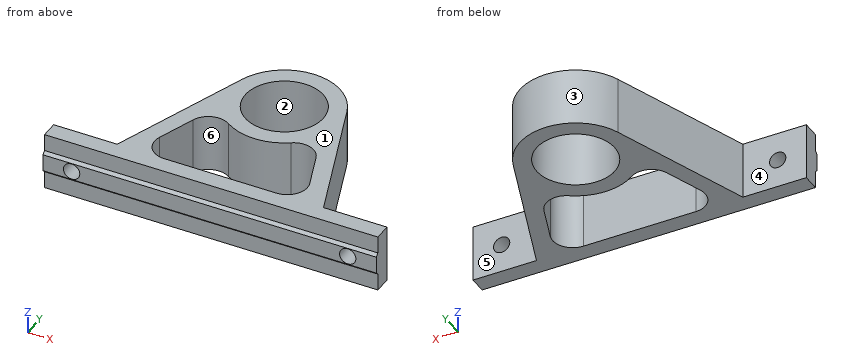
```python
from build123d import *

# Parameters (mm, degrees)
F0_R        = 13.6
F0_W        = 59.3062995352
F0_H        = 6
F1_DEPTH    = 20
F2_R        = 7
F3_W        = 116.4440756161
F3_H        = 2
F4_DEPTH    = 1
F5_T4_DEPTH = 116.4440756161
F5_T9_DEPTH = 116.4440756161
F6_R        = 2.85
F7_DEPTH    = 25


# Not quite as in the source:
# - a fillet or chamfer that OpenCascade refuses, or shapes differently, is made with other operations: its cross-section is extruded or revolved along the edge and cut away or added


with BuildPart() as f1:
    # F0 (on Top) → F1 (new body)
    with BuildSketch(Plane.XY):
        with BuildLine():
            ThreePointArc((17.4985003919, 39.3946247011), (18.9930350082, 43.5824643545), (19.5, 48))
            ThreePointArc((19.5, 48), (19.2037511837, 51.3861394645), (18.3240061053, 54.6693927949))
            ThreePointArc((18.3240061053, 54.6693927949), (0, 67.5), (-18.3240061053, 54.6693927949))
            ThreePointArc((-18.3240061053, 54.6693927949), (-19.4715851439, 46.9476825647), (-17.4985003919, 39.3946247011))
            ThreePointArc((-17.4985003919, 39.3946247011), (0, 28.5), (17.4985003919, 39.3946247011))
        make_face()
        with Locations((0, 48)):
            Circle(F0_R, mode=Mode.SUBTRACT)
        with BuildLine():
            ThreePointArc((-17.4985003919, 39.3946247011), (-19.4715851439, 46.9476825647), (-18.3240061053, 54.6693927949))
            Line((-18.3240061053, 54.6693927949), (-36.0382164025, 6))
            Line((-36.0382164025, 6), (-29.6531497676, 6))
            Line((-29.6531497676, 6), (-17.4985003919, 39.3946247011))
        make_face()
        Polygon((-29.6531497676, 6), (-36.0382164025, 6), (-38.2220378081, 0), (-29.6531497676, 0), align=None)
        Polygon((-38.2220378081, 0), (-36.0382164025, 6), (-58.2220378081, 6), (-58.2220378081, 0), align=None)
        with Locations((0, 3)):
            Rectangle(F0_W, F0_H)
        Polygon((38.2220378081, 0), (36.0382164025, 6), (29.6531497676, 6), (29.6531497676, 0), align=None)
        Polygon((58.2220378081, 6), (36.0382164025, 6), (38.2220378081, 0), (58.2220378081, 0), align=None)
        with BuildLine():
            ThreePointArc((18.3240061053, 54.6693927949), (19.2037511837, 51.3861394645), (19.5, 48))
            ThreePointArc((19.5, 48), (18.9930350082, 43.5824643545), (17.4985003919, 39.3946247011))
            Line((17.4985003919, 39.3946247011), (29.6531497676, 6))
            Line((29.6531497676, 6), (36.0382164025, 6))
            Line((36.0382164025, 6), (18.3240061053, 54.6693927949))
        make_face()
    extrude(amount=F1_DEPTH)

    # F2
    f2_edges = [f1.edges().sort_by_distance(p)[0] for p in [
        (-17.4985, 39.394625, 10),
        (17.4985, 39.394625, 10),
        (-29.65315, 6, 10),
        (29.65315, 6, 10),
    ]]
    fillet(f2_edges, radius=F2_R)

    # F3 (on face) → F4 (join)
    with BuildSketch(Plane.XZ):
        with Locations((0, 10)):
            Rectangle(F3_W, F3_H)
    extrude(amount=F4_DEPTH)

    # F5: chamfer of 3 on 2 edges, made by hand


with BuildPart() as f5_tool2:
    # F5_s3 → F5_t4 (new body)
    with BuildSketch(Plane.YZ.offset(58.2220378081)):
        Polygon((0, 14), (-3, 11), (0, 11), align=None)
    extrude(amount=-F5_T4_DEPTH)

    split(bisect_by=Plane.XZ.offset(1), keep=Keep.BOTTOM)


with BuildPart() as f1_1:
    add(f1.part)

    # F5_t1: union F5_tool2
    add(f5_tool2.part)


with BuildPart() as f5_tool7:
    # F5_s8 → F5_t9 (new body)
    with BuildSketch(Plane.YZ.offset(-58.2220378081)):
        Polygon((0, 6), (-3, 9), (0, 9), align=None)
    extrude(amount=F5_T9_DEPTH)

    split(bisect_by=Plane.XZ.offset(1), keep=Keep.BOTTOM)


with BuildPart() as f1_2:
    add(f1_1.part)

    # F5_t6: union F5_tool7
    add(f5_tool7.part)

    # F6 (on face) → F7 (cut)
    with BuildSketch(Plane(origin=(0, 6, 0), x_dir=(-1, 0, 0), z_dir=(0, 1, 0))):
        with Locations((48.2220378081, 10)):
            Circle(F6_R)
        with Locations((-48.2220378081, 10)):
            Circle(F6_R)
    extrude(amount=-F7_DEPTH, mode=Mode.SUBTRACT)


solid = f1_2.part
```
Read the model definition and answer for the solid it produces. Units are mm, in the model's axes. Face numbers are marked on the shaded views. A direction names the side the tool comes from. Coordinates: 2 decimals unless noted, no trailing zeros. Write each loop counter-clockwise with the first axis right and the second up, starting at its lowest first coordinate (ties: lowest second). Pieces come first, ordered by that corner, then holes. Notation, with made-up numbers: (-29, 57) -> (1, 57) arc R21 ccw to (1, 91) -> close; hole circle Ø11 at (-10, 48). An arc over 180 degrees is marked (long way). Write item = value, one per line.
(1) Section D-D on x = 37.5 is taken. Write down the section's boundary in (y, z), plus the area to 3 significant figures.
From the geometry:
outline = (-1, 7) -> (0, 6) -> (0, 0) -> (6, 0) -> (6, 20) -> (0, 20) -> (0, 14) -> (-1, 13) -> close
area = 127 mm2
(2) Section A-A on y = 4 is taken. Write down the section's boundary in (x, z), plus the area to 3 significant figures.
From the geometry:
outline = (-58.22, 0) -> (58.22, 0) -> (58.22, 20) -> (-58.22, 20) -> close; hole circle Ø5.7 at (-48.22, 10); hole circle Ø5.7 at (48.22, 10)
area = 2,280 mm2
(3) Which of the six approach directions +Z, -Z, +X, -X, +Y, -Y give full straight-line access (tool end or side, diameter ignored) to the marked faces 4, 5 and 6?
From the geometry:
face_4 = +Z, -Z, -X, +Y
face_5 = +Z, -Z, +X, +Y
face_6 = +Z, -Z
(4) Given pin 1 Ø8 at (y, z) = (55.5, 5.5) entering from -X; pin 2 Ø8 at (y, z) = (34.5, 15) entering from -X; pin 3 Ø3 at (x, z) = (28.5, 17.5) entering from -Y; pin 4 Ø24.5 at (x, y) = (0, 48) entering from -Z, each flat-ended and moving along its own axis, determine where each tip first touches the part or whether it passes through.
From the geometry:
pin_1 = -19.48
pin_2 = -27.12
pin_3 = 0
pin_4 = through
(5) Section C-C on y = 53.5 is taken. Write down the section's boundary in (x, z).
From the geometry:
outline = (-18.75, 0) -> (-12.44, 0) -> (-12.44, 20) -> (-18.75, 20) -> close; (12.44, 0) -> (18.75, 0) -> (18.75, 20) -> (12.44, 20) -> close
(6) Section B-B on x = 0 is taken. Write down the section's boundary in (y, z).
From the geometry:
outline = (-1, 7) -> (0, 6) -> (0, 0) -> (6, 0) -> (6, 20) -> (0, 20) -> (0, 14) -> (-1, 13) -> close; (28.5, 0) -> (34.4, 0) -> (34.4, 20) -> (28.5, 20) -> close; (61.6, 0) -> (67.5, 0) -> (67.5, 20) -> (61.6, 20) -> close
(7) Straight lines are drawn through the part: L1, parallel to Y at x = 7.5, z = 7.75; L2, parallel to Y at x = -50, z = 5.75; L3, parallel to Y at x = -8, z = 13.5. For each, find the intervals that lie inside material, in ascending order. Write a range as from..to.
From the geometry:
L1 = -1..6, 30..36.65, 59.35..66
L2 = 0..6
L3 = -0.5..6, 30.22..37, 59..65.78
(8) For a pull along X with two mould halves and no side action, classify the marked faces 1, 2 and 3 as +X half, -X half, draft (parallel to the pull), parting line (faces both ways), or undercut.
From the geometry:
face_1 = draft
face_2 = undercut
face_3 = parting line
